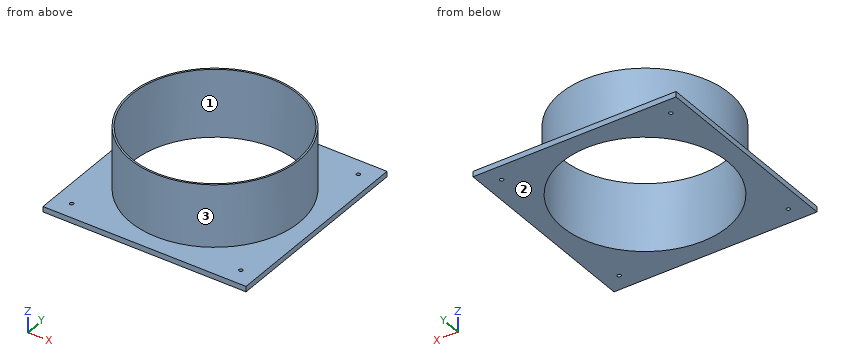
from build123d import *

# Parameters (mm, degrees)
F0_W     = 120
F0_H     = 120
F0_R     = 1.1
F0_R_2   = 50
F1_DEPTH = 3.2
F0_R_3   = 49
F2_DEPTH = 40


with BuildPart() as f1:
    # F0 (on Top) → F1 (new body)
    with BuildSketch(Plane.XY):
        Rectangle(F0_W, F0_H)
        with Locations((-50, -50)):
            Circle(F0_R, mode=Mode.SUBTRACT)
        with Locations((50, -50)):
            Circle(F0_R, mode=Mode.SUBTRACT)
        with Locations((-50, 50)):
            Circle(F0_R, mode=Mode.SUBTRACT)
        Circle(F0_R_2, mode=Mode.SUBTRACT)
        with Locations((50, 50)):
            Circle(F0_R, mode=Mode.SUBTRACT)
    extrude(amount=F1_DEPTH)

    # F0 (on Top) → F2 (join)
    with BuildSketch(Plane.XY):
        Circle(F0_R_2)
        Circle(F0_R_3, mode=Mode.SUBTRACT)
    extrude(amount=F2_DEPTH)


solid = f1.part
Check sheet for the modelled part. Datum: model origin and axes. Units: mm. Face numbers are marked on the shaded views. Round coordinates to 2 decimals unless told otherwise and drop trailing zeros. Loops run counter-clockwise (first coordinate to the right, second up) from the corner with the lowest first, then second, coordinate; pieces in that order, holes last. Notation, with made-up numbers: M -9,12 L 33,12 A18 cw 33,43 Z; hole C -0.75,82 d10. An arc over 180 degrees is marked long. One line per item, written item: value.
(1) Release check for a two-part mould opening along Y. For the marked faces 1, 2 and 3 record: +Y half, -Y half, draft (parallel to the pull), parting line (faces both ways), or undercut.
Computed values:
face 1: undercut
face 2: draft
face 3: parting line
(2) Sectioned sample at A-A, the plane x = 0. Record the cut outline in (y, z), then the cut area to 3 significant figures.
Computed values:
outline: M -60,0 L -49,0 L -49,40 L -50,40 L -50,3.2 L -60,3.2 Z; M 49,0 L 60,0 L 60,3.2 L 50,3.2 L 50,40 L 49,40 Z
area: 144 mm^2
(3) Thickness scan on line 1 (Y direction, x = -50, z = 1.4); line 2 (Z direction, x = 46, y = 30.5); line 3 (Y direction, x = -0.5, z = 38). Record the ranges inside material, lowest first.
Computed values:
line 1: y = -60 to -51.1, -48.9 to 48.9, 51.1 to 60
line 2: z = 0 to 3.2
line 3: y = -50 to -49, 49 to 50
(4) Depth check by flat-ended pin: pin 1 Ø10 at (x, z) = (5.5, 17.5) entering from +Y; pin 2 Ø6 at (y, z) = (40, 16) entering from +X; pin 3 Ø3 at (x, z) = (31.5, 32) entering from +Y. Enter the tip coordinate at first touch or a pass-through.
Computed values:
pin 1: stops at y = 50
pin 2: stops at x = 33.63
pin 3: stops at y = 40
(5) Sectioned sample at C-C, the plane z = 22.5. Record the cut outline in (x, y), then the cut area to 3 significant figures.
Computed values:
outline: C 0,0 d100; hole C 0,0 d98
area: 311 mm^2
